For this review, take the finished solid that the model builds, in its own axes (mm). A direction names the side the tool comes from. Coordinates: 2 decimals unless noted, no trailing zeros. Write each loop counter-clockwise with the first axis right and the second up, starting at its lowest first coordinate (ties: lowest second). Pieces come first, ordered by that corner, then holes. Notation, with made-up numbers: M 50.5,63.5 L 74.5,63.5 A24 cw 74.5,74.5 Z; hole C 23,-23 d8. An arc over 180 degrees is marked long. One line per question, with ' | ' between items.
from build123d import *

# Parameters (mm, degrees)
SKETCH1_W           = 247.5
SKETCH1_H           = 115
BOSS_EXTRUDE1_DEPTH = 20
SKETCH2_R           = 4.4
CUT_EXTRUDE1_DEPTH  = 17.5
SKETCH3_R           = 4.4
CUT_EXTRUDE2_DEPTH  = 17.5
SKETCH6_W           = 10
SKETCH6_H           = 70
BOSS_EXTRUDE3_DEPTH = 20
SKETCH7_W           = 15
SKETCH7_H           = 60
CUT_EXTRUDE4_DEPTH  = 20


with BuildPart() as part:
    # Sketch1 → Boss-Extrude1 (new body)
    with BuildSketch(Plane(origin=(0, 0, 0), x_dir=(0, 0, -1), z_dir=(1, 0, 0))):
        Rectangle(SKETCH1_W, SKETCH1_H)
    extrude(amount=BOSS_EXTRUDE1_DEPTH)

    # Sketch2 → Cut-Extrude1 (cut)
    with BuildSketch(Plane(origin=(0, 57.5, 0), x_dir=(1, 0, 0), z_dir=(0, 1, 0))):
        with Locations((10, -113.75)):
            Circle(SKETCH2_R)
    extrude(amount=-CUT_EXTRUDE1_DEPTH, mode=Mode.SUBTRACT)

    # Sketch3 → Cut-Extrude2 (cut)
    with BuildSketch(Plane.XZ.offset(57.5)):
        with Locations((10, 113.75)):
            Circle(SKETCH3_R)
    extrude(amount=-CUT_EXTRUDE2_DEPTH, mode=Mode.SUBTRACT)

    # Sketch6 → Boss-Extrude3 (add)
    with BuildSketch(Plane(origin=(20, 0, 0), x_dir=(0, 0, -1), z_dir=(1, 0, 0))):
        with Locations((103.75, 0)):
            Rectangle(SKETCH6_W, SKETCH6_H)
    extrude(amount=BOSS_EXTRUDE3_DEPTH)

    # Sketch7 → Cut-Extrude4 (cut)
    with BuildSketch(Plane(origin=(0, 0, -108.75), x_dir=(-1, 0, 0), z_dir=(0, 0, -1))):
        with Locations((-27.5, 0)):
            Rectangle(SKETCH7_W, SKETCH7_H)
    extrude(amount=-CUT_EXTRUDE4_DEPTH, mode=Mode.SUBTRACT)


solid = part.part
1. Draft analysis for pull direction Y (two halves, no side actions). For faces 1 (the cylindrical face through (9.046, 48.872, 118.045)), 2 (the flat face through (35, 0, -104)), 3 (the flat face through (10, -40, 114)), state which applies: pulls with the +Y half, pulls with the -Y half, needs draft (parallel to the pull), parting line crosses it, or undercut.
Computed values:
face 1: needs draft | face 2: undercut | face 3: pulls with the -Y half
2. Take a section at A-A on y = -21. State the section outline as (x, z) points.
Computed values:
outline: M 0,-123.75 L 20,-123.75 L 20,123.75 L 0,123.75 Z; M 35,-108.75 L 40,-108.75 L 40,-98.75 L 35,-98.75 Z
3. Take a section at C-C on z = -85. State the section outline as (x, y) points.
Computed values:
outline: M 0,-57.5 L 20,-57.5 L 20,57.5 L 0,57.5 Z
4. For line 1 along Z through (x, y) = (10, -45.5); line 2 along X through (y, z) = (52.25, 113.75); line 3 along X through (y, z) = (-26, -23.5), list the stretches that pass through material, from the lowest coordinate up.
Computed values:
line 1: z = -123.75 to 109.35, 118.15 to 123.75 | line 2: x = 0 to 5.6, 14.4 to 20 | line 3: x = 0 to 20
5. Clearance check with flat-ended pins moving along their axes: P1, Ø1, axis at y = -27, z = 1.5, coming from the -X side; P2, Ø6, axis at x = 34, y = 40, coming from the +Z side; P3, Ø12, axis at y = -25.5, z = 85, coming from the +X side; P4, Ø5, axis at x = 34, z = -104, coming from the +Y side. State where each tip first meets the part, or that it passes through.
Computed values:
P1: stops at x = 0 | P2: passes through | P3: stops at x = 20 | P4: stops at y = 35
6. Machinability: for faces 4 (the cylindrical face through (9.046, -48.872, 109.455)), 5 (the flat face through (30, 35, -104)), 6 (the flat face through (28, 30, -104)), 7 (the flat face through (37, 0, -98.75)), which of the approach directions +Z, -Z, +X, -X, +Y, -Y give a long, thin tool a straight path to every point of the face, cutting with its end or side? Answer none if there is none.
Computed values:
face 4: -Y | face 5: +Z, -Z, +X, +Y | face 6: +Z, -Z | face 7: +Z, +X, +Y, -Y
7. Take a section at B-B on x = 27. State the section outline as (y, z) points.
Computed values:
outline: M -35,-108.75 L -30,-108.75 L -30,-98.75 L -35,-98.75 Z; M 30,-108.75 L 35,-108.75 L 35,-98.75 L 30,-98.75 Z
